Build history of the part. All positions in model axes, mm. A direction names the side the tool comes from. Give positions to 0.01 mm unless a question says otherwise; leave off trailing zeros. Write each loop counter-clockwise with the first axis right and the second up, starting at its lowest first coordinate (ties: lowest second). Pieces come first, ordered by that corner, then holes. Notation, with made-up numbers: M -27,8 L -1,8 A14 cw -1,24 Z; hole C 11,16 d11. An arc over 180 degrees is marked long. Return JSON: item names as keys, results as strings. Group by question number.
Q1. Tool access for faces 5 (the flat face through (38.17, 3, 2)), 6 (the flat face through (41.345, 7, 2)), 7 (the flat face through (39.736, 9.041, 1.565)), 8 (the flat face through (19, 31.752, 2)), 9 (the flat face through (39.736, 26.451, 1.565)): list every direction of +Z, -Z, +X, -X, +Y, -Y with a clear straight run to the whole face (end or side of a thin tool).
Q2. Band-saw the part on C-C, the plane y = 11. Give the cut face in (x, z) (3 decimals), then the cut area to 3 significant figures.
Q3. Flat gauge pins, fed straight in: pin 1 Ø1 at (y, z) = (19.5, 1.5) entering from +X; pin 2 Ø1.5 at (x, y) = (22, 3.5) entering from -Z; pin 3 Ø1 at (y, z) = (2, 1) entering from -X; pin 4 Ø3 at (x, y) = (19.09, 7.14) entering from -Z. Where does each tip first touch, or does it go through?
Q4. Band-saw the part on B-B, the plane z = 1.05. Count the separate pieces of the cut face and the enclosed holes in it, then the cut area to 3 significant figures.
Q5. Band-saw the part on A-A, the plane y = 6.5. Give the cut face in (x, z) (3 decimals), then the cut area to 3 significant figures.
Q6. Pull direction X, two halves, no side cores. Call faces 1 (the flat face through (-3.175, 7, 2)), 2 (the flat face through (41.345, 25, 2)), 3 (the flat face through (0, 29, 2)), 4 (the flat face through (19, 16, 3.175)): +X half, -X half, draft (parallel to the pull), parting line (faces both ways), or undercut.
Q7. Wall check: probe 1 along X at (y, z) = (13, 1.1); probe 2 along Y at (x, z) = (18, 1.35); probe 3 along X at (y, z) = (7, 1.7) (3 decimals). Give the ranges that are in metal, low to high.
from build123d import *

# Parameters (mm, degrees)
SKETCH1_W           = 38.170316933
SKETCH1_H           = 31.751666379
BOSS_EXTRUDE1_DEPTH = 3.175
SKETCH2_R           = 3.175
SKETCH2_R_2         = 1.5875
CUT_EXTRUDE1_DEPTH  = 3.175


with BuildPart() as part:
    # Sketch1 → Boss-Extrude1 (new body)
    with BuildSketch(Plane.XY):
        with Locations((19.085158467, 15.87583319)):
            Rectangle(SKETCH1_W, SKETCH1_H)
        Polygon((-3.175, 24.607083189), (-3.175, 27.147083189), (0, 25.774124793), (0, 23.337083189), (-3.175, 22.067083189), align=None)
        Polygon((-3.175, 7.144583189), (-3.175, 9.684583189), (0, 8.414583189), (0, 5.977541585), (-3.175, 4.604583189), align=None)
        Polygon((41.345316933, 7.144583189), (41.345316933, 4.604583189), (38.170316933, 5.977541585), (38.170316933, 8.414583189), (41.345316933, 9.684583189), align=None)
        Polygon((41.345316933, 24.607083189), (41.345316933, 22.067083189), (38.170316933, 23.337083189), (38.170316933, 25.774124793), (41.345316933, 27.147083189), align=None)
    extrude(amount=BOSS_EXTRUDE1_DEPTH)

    # Sketch2 → Cut-Extrude1 (cut)
    with BuildSketch(Plane.XY.offset(3.175)):
        with Locations((19.085158466, 24.607083189)):
            Circle(SKETCH2_R)
        with Locations((19.085158466, 7.144583189)):
            Circle(SKETCH2_R_2)
    extrude(amount=-CUT_EXTRUDE1_DEPTH, mode=Mode.SUBTRACT)


solid = part.part
From the geometry:
{
 "1": {"face 5": "+Z, -Z, -Y", "face 6": "+Z, -Z, +X, +Y, -Y", "face 7": "+Z, -Z", "face 8": "+Z, -Z, +X, -X, +Y", "face 9": "+Z, -Z, +Y"},
 "2": {"outline": "M 0,0 L 38.17,0 L 38.17,3.175 L 0,3.175 Z", "area": "121 mm^2"},
 "3": {"pin 1": "stops at x = 38.17", "pin 2": "stops at z = 0", "pin 3": "stops at x = 0", "pin 4": "passes through"},
 "4": {"separate pieces": "1", "enclosed holes": "2", "area": "1,220 mm^2"},
 "5": {"outline": "M -3.175,0 L 17.634,0 L 17.634,3.175 L -3.175,3.175 Z; M 20.536,0 L 41.345,0 L 41.345,3.175 L 20.536,3.175 Z", "area": "132 mm^2"},
 "6": {"face 1": "-X half", "face 2": "+X half", "face 3": "undercut", "face 4": "draft"},
 "7": {"probe 1": "x = 0 to 38.17", "probe 2": "y = 0 to 5.99, 8.3 to 21.62, 27.59 to 31.75", "probe 3": "x = -3.175 to 17.504, 20.666 to 41.345"}
}
